Geometry: final body of the model. Coordinates: model frame, mm. A direction names the side the tool comes from. Coordinates: 2 decimals unless noted, no trailing zeros. Order: outer loops, then holes, each group sorted by start corner. A loop starts at its lowest first (then second) coordinate and runs counter-clockwise, first axis right, second up. Notation, with made-up numbers: (56, -26.5) - (95, -26.5) arc R24 ccw to (95, 2.5) - close; hole circle Ø9 at (24, 50). An arc over 180 degrees is marked (long way). Use a Markdown table: item, result. Add a question column.
```python
from build123d import *

# Parameters (mm, degrees)
BOSS_EXTRU_1_DEPTH      = 30
ENL_V_MAT_EXTRU_1_DEPTH = 31
ENL_V_MAT_EXTRU_2_DEPTH = 25
ESQUISSE4_R             = 3
ENL_V_MAT_EXTRU_3_DEPTH = 5
CONG_1_R                = 1


with BuildPart() as part:
    # Esquisse1 → Boss.-Extru.1 (new body)
    with BuildSketch(Plane.XY):
        with BuildLine():
            Line((-55, 0), (55, 0))
            Line((55, 0), (55, 5))
            Line((55, 5), (37.55, 5))
            Line((37.55, 5), (37.55, 32.55))
            ThreePointArc((37.55, 32.55), (0, 70.1), (-37.55, 32.55))
            Line((-37.55, 32.55), (-37.55, 5))
            Line((-37.55, 5), (-55, 5))
            Line((-55, 5), (-55, 0))
        make_face()
    extrude(amount=BOSS_EXTRU_1_DEPTH)

    # Esquisse2 → Enlèv. mat.-Extru.1 (cut, through all)
    with BuildSketch(Plane(origin=(0, 0, 0), x_dir=(-1, 0, 0), z_dir=(0, 0, -1))):
        with BuildLine():
            Line((-22.5, 32.55), (-22.5, 0))
            Line((-22.5, 0), (22.5, 0))
            Line((22.5, 0), (22.5, 32.55))
            ThreePointArc((22.5, 32.55), (0, 55.05), (-22.5, 32.55))
        make_face()
    extrude(amount=-ENL_V_MAT_EXTRU_1_DEPTH, mode=Mode.SUBTRACT)

    # Esquisse3 → Enlèv. mat.-Extru.2 (cut)
    with BuildSketch(Plane(origin=(0, 0, 0), x_dir=(-1, 0, 0), z_dir=(0, 0, -1))):
        with BuildLine():
            Line((-32.55, 32.55), (-32.55, 0))
            Line((-32.55, 0), (32.55, 0))
            Line((32.55, 0), (32.55, 32.55))
            ThreePointArc((32.55, 32.55), (0, 65.1), (-32.55, 32.55))
        make_face()
    extrude(amount=-ENL_V_MAT_EXTRU_2_DEPTH, mode=Mode.SUBTRACT)

    # Esquisse4 → Enlèv. mat.-Extru.3 (cut)
    with BuildSketch(Plane.XZ):
        with Locations((47.5, 7.5)):
            Circle(ESQUISSE4_R)
        with Locations((-47.5, 7.5)):
            Circle(ESQUISSE4_R)
        with Locations((47.5, 22.5)):
            Circle(ESQUISSE4_R)
        with Locations((-47.5, 22.5)):
            Circle(ESQUISSE4_R)
    extrude(amount=-ENL_V_MAT_EXTRU_3_DEPTH, mode=Mode.SUBTRACT)

    # Congé1
    cong_1_edges = [part.edges().sort_by_distance(p)[0] for p in [
        (-37.55, 5, 15),
        (37.55, 5, 15),
    ]]
    fillet(cong_1_edges, radius=CONG_1_R)


solid = part.part
```
1) Section query C-C (y = 12). Return the cut outline in (x, z), and give its area (4 significant figures).
2) Draft query along X for faces 1 (the flat face through (-22.5, 16, 27)), 2 (the flat face through (-47, 5, 15)), 3 (the flat face through (-32.55, 16, 12)), 4 (the flat face through (37.55, 19, 15)). Return one class per face: released by +X, released by -X, zero draft, split by the parting line, or undercut.
3) Line query: line 1 (Z direction, x = -47.5, y = 2.7); line 2 (X direction, y = 11.5, z = 27); line 3 (X direction, y = 9, z = 10.5). Output: solid intervals per line, ascending. Write a range as from..to.
4) Section query B-B (z = 7.5). Return the cut outline in (x, y), and give its area (3 significant figures).
5) Section query D-D (x = 0). Return the cut outline in (y, z).
6) First-contact query: pin 1 (13.5 mm diameter, centred on y = 19, z = 8, fed in from +X); pin 2 (8 mm diameter, centred on x = -47.5, z = 7.5, fed in from +Y); pin 3 (12 mm diameter, centred on x = -28, z = 12.5, fed in from +Y); pin 4 (7 mm diameter, centred on x = -47.5, z = 22.5, fed in from -Y). Flat tips, straight axial feed; report the tip coordinate or a pass-through.
7) Section query A-A (x = 47.5). Return the cut outline in (y, z), and give its area (3 significant figures).
8) Access query for faces 5 (the flat face through (-37.55, 19, 15)), 6 (the cylindrical face through (-0.716, 65.092, 12.325)), 7 (the flat face through (47, 5, 15)), 8 (the flat face through (22.5, 17, 27)). Directions: +Z, -Z, +X, -X, +Y, -Y. A direction counts if a zero-diameter tool reaches every point of the face in a straight line with its end or side. Return the directions, or none.
From the geometry:
| question | item | result |
|---|---|---|
| 1 | outline | (-37.55, 0) - (-32.55, 0) - (-32.55, 25) - (-22.5, 25) - (-22.5, 30) - (-37.55, 30) - close; (22.5, 25) - (32.55, 25) - (32.55, 0) - (37.55, 0) - (37.55, 30) - (22.5, 30) - close |
| 1 | area | 400.5 mm^2 |
| 2 | face 1 | undercut |
| 2 | face 2 | zero draft |
| 2 | face 3 | undercut |
| 2 | face 4 | released by +X |
| 3 | line 1 | z = 0..4.5, 10.5..19.5, 25.5..30 |
| 3 | line 2 | x = -37.55..-22.5, 22.5..37.55 |
| 3 | line 3 | x = -37.55..-32.55, 32.55..37.55 |
| 4 | outline | (-55, 0) - (-50.5, 0) - (-50.5, 5) - (-55, 5) - close; (-44.5, 0) - (-32.55, 0) - (-32.55, 32.55) arc R32.55 cw to (32.55, 32.55) - (32.55, 0) - (44.5, 0) - (44.5, 5) - (38.55, 5) arc R1 cw to (37.55, 6) - (37.55, 32.55) arc R37.55 ccw to (-37.55, 32.55) - (-37.55, 6) arc R1 cw to (-38.55, 5) - (-44.5, 5) - close; (50.5, 0) - (55, 0) - (55, 5) - (50.5, 5) - close |
| 4 | area | 991 mm^2 |
| 5 | outline | (55.05, 25) - (65.1, 25) - (65.1, 0) - (70.1, 0) - (70.1, 30) - (55.05, 30) - close |
| 6 | pin 1 | stops at x = 37.55 |
| 6 | pin 2 | stops at y = 5 |
| 6 | pin 3 | stops at y = 62.98 |
| 6 | pin 4 | stops at y = 0 |
| 7 | outline | (0, 0) - (5, 0) - (5, 4.5) - (0, 4.5) - close; (0, 10.5) - (5, 10.5) - (5, 19.5) - (0, 19.5) - close; (0, 25.5) - (5, 25.5) - (5, 30) - (0, 30) - close |
| 7 | area | 90.0 mm^2 |
| 8 | face 5 | +Z, -Z, -X, +Y |
| 8 | face 6 | -Z, -Y |
| 8 | face 7 | +Z, -Z, +X, +Y |
| 8 | face 8 | +Z, -Z, -Y |
